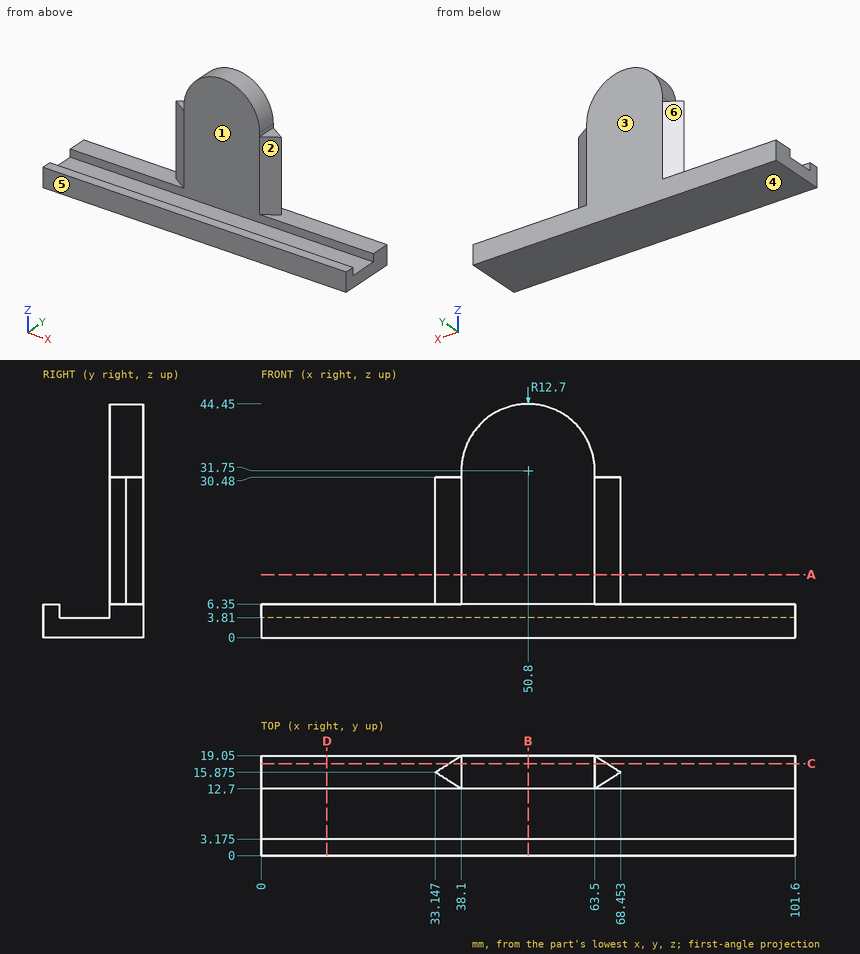
Part print with two shaded views. Sizes in mm from the minimum x, y, z corner. A direction names the side the tool comes from. Round coordinates to 2 decimals unless told otherwise and drop trailing zeros. Write each loop counter-clockwise with the first axis right and the second up, starting at its lowest first coordinate (ties: lowest second). Pieces come first, ordered by that corner, then holes. Notation, with made-up numbers: M 73,49 L 122,49 A15 ccw 122,56 Z; hole C 26.5,20 d9. An arc over 180 degrees is marked long. Put each result on its own line as item: value. Start each with the question number.
1) 3-axis set-ups, long thin cutter, end or side, ignore diameter. For the marked faces 5 and 6: which of +Z, -Z, +X, -X, +Y, -Y reach the whole face in a straight line?
2) Saw through at A-A, the plane z = 12. Write the cut outline in (x, y) (3 decimals), and give its area (3 significant figures).
3) Saw through at C-C, the plane y = 17.5. Write the cut outline in (x, z), and give its area (3 significant figures).
4) Saw through at B-B, the plane x = 50.8. Write the cut outline in (y, z) (3 decimals).
5) Pull direction Y, two halves, no side cores. Call the marked faces 1, 2, 3 and 4: pulls with the +Y half, pulls with the -Y half, needs draft (parallel to the pull), parting line crosses it, or undercut.
6) Pin check, flat tips, straight feed: pin 1 Ø1 at (y, z) = (13, 23.5) entering from -X; pin 2 Ø2.5 at (x, y) = (56, 1.5) entering from +Z; pin 3 Ø1.4 at (y, z) = (16, 31) entering from -X; pin 4 Ø6 at (x, y) = (26.5, 2.5) entering from -Z. Stop position of each tip, or through.
7) Drill centre lines: probe 1 along Y at (x, z) = (76, 6) (3 decimals); probe 2 along Z at (x, y) = (93, 14.75); probe 3 along Z at (x, y) = (66, 3.5). Where is each one in solid material? Low to high. Write a range as [from, to].
8) Saw through at D-D, the plane x = 12.5. Write the cut outline in (y, z) (3 decimals).
Resolved:
1. face 5: +Z, -Z, +X, -X, -Y
1. face 6: +Z, -X, +Y
2. outline: M 33.147,15.875 L 38.1,12.7 L 63.5,12.7 L 68.453,15.875 L 63.5,19.05 L 38.1,19.05 Z
2. area: 193 mm²
3. outline: M 0,0 L 101.6,0 L 101.6,6.35 L 65.92,6.35 L 65.92,30.48 L 63.5,30.48 L 63.5,31.75 A12.7 ccw 38.1,31.75 L 38.1,30.48 L 35.68,30.48 L 35.68,6.35 L 0,6.35 Z
3. area: 1,660 mm²
4. outline: M 0,0 L 19.05,0 L 19.05,44.45 L 12.7,44.45 L 12.7,3.81 L 3.175,3.81 L 3.175,6.35 L 0,6.35 Z
5. face 1: undercut
5. face 2: pulls with the -Y half
5. face 3: pulls with the +Y half
5. face 4: needs draft
6. pin 1: x = 36.85
6. pin 2: z = 6.35
6. pin 3: x = 33.15
6. pin 4: z = 0
7. probe 1: [0, 3.175], [12.7, 19.05]
7. probe 2: [0, 6.35]
7. probe 3: [0, 3.81]
8. outline: M 0,0 L 19.05,0 L 19.05,6.35 L 12.7,6.35 L 12.7,3.81 L 3.175,3.81 L 3.175,6.35 L 0,6.35 Z
